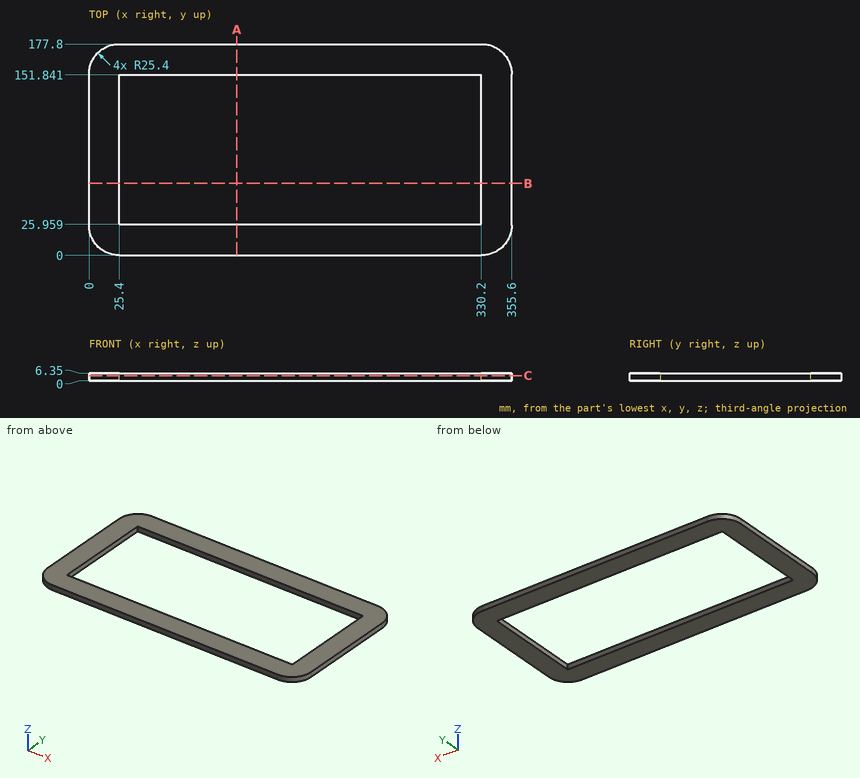
Answer from the drawing. Dimensions are ordinates in mm from the lowest x, y and z of the part. Coordinates: 2 decimals unless noted, no trailing zeros. Write each loop counter-clockwise with the first axis right and the second up, starting at its lowest first coordinate (ties: lowest second). Pieces come first, ordered by that corner, then holes. Notation, with made-up numbers: M -28.5,73 L 29.5,73 A25 cw 29.5,90 Z; hole C 42,-6 d5. An arc over 180 degrees is marked long. Put each result on its own line as item: value. Start each with the question number.
1. A cutting plane is placed at C-C on z = 4.5. Write down the section's boundary in (x, y), then the cut area to 3 significant figures.
2. A cutting plane is placed at B-B on y = 60.5. Write down the section's boundary in (x, z).
3. A cutting plane is placed at A-A on x = 124.5. Write down the section's boundary in (y, z), then the cut area to 3 significant figures.
4. Consider line 1 (X direction, y = 26.5, z = 4); line 2 (Y direction, x = 75.5, z = 5.75); line 3 (Y direction, x = 331.5, z = 2.5). Determine where each line is inside the solid, lowest interval first. Write a range as from..to.
Resolved:
1. outline: M 0,25.4 A25.4 ccw 25.4,0 L 330.2,0 A25.4 ccw 355.6,25.4 L 355.6,152.4 A25.4 ccw 330.2,177.8 L 25.4,177.8 A25.4 ccw 0,152.4 Z; hole M 25.4,25.96 L 330.2,25.96 L 330.2,151.84 L 25.4,151.84 Z
1. area: 24,300 mm2
2. outline: M 0,0 L 25.4,0 L 25.4,6.35 L 0,6.35 Z; M 330.2,0 L 355.6,0 L 355.6,6.35 L 330.2,6.35 Z
3. outline: M 0,0 L 25.96,0 L 25.96,6.35 L 0,6.35 Z; M 151.84,0 L 177.8,0 L 177.8,6.35 L 151.84,6.35 Z
3. area: 330 mm2
4. line 1: x = 0..25.4, 330.2..355.6
4. line 2: y = 0..25.96, 151.84..177.8
4. line 3: y = 0.03..177.77
